Design review of the part built by this model. Coordinates are the model's own, in mm. Face numbers are marked on the shaded views. A direction names the side the tool comes from. Give positions to 0.01 mm unless a question says otherwise; leave off trailing zeros. Loops run counter-clockwise (first coordinate to the right, second up) from the corner with the lowest first, then second, coordinate; pieces in that order, holes last. Notation, with made-up numbers: (31.5, 34) -> (81.5, 34) arc R6 ccw to (81.5, 39) -> close; hole circle Ø5 at (-17, 46). An arc over 180 degrees is marked (long way). Answer in a Markdown table with one row per item. Add a question column.
(1) Consider section C-C on x = 121.5. Write out the cut boundary in (y, z).
(2) Draft analysis for pull direction Z (two halves, no side actions). For the marked faces 4, 5, 6 and 7, state which applies: +Z half, -Z half, draft (parallel to the pull), parting line (faces both ways), or undercut.
(3) Consider section B-B on z = -53. Write out the cut boundary in (x, y), then the cut area to 3 significant figures.
(4) Consider section D-D on z = -91. Write out the cut boundary in (x, y).
(5) For pin 1 (3 mm diameter, centred on x = 25, z = -34, fed in from -Y); pin 2 (4.5 mm diameter, centred on x = 77, y = -2.5, fed in from -Z); pin 3 (6.5 mm diameter, centred on x = 144, z = -50.5, fed in from +Y), all flat-tipped, find the tip position at first contact; note any pin that passes through.
(6) For the marked faces 1, 2 and 3, list the 3-axis set-ups (+Z, -Z, +X, -X, +Y, -Y) from which the entire face can be reached by the end or side of a thin tool; tool diameter is ignored.
(7) For line 1 (Y direction, x = 143.5, z = -72.5); line 2 (Z direction, x = 125.5, y = 10); line 3 (Y direction, x = 27.5, z = -44), list the stretches that pass through material, from the lowest coordinate up.
Autodesk Fusion 360 part; units mm, degrees
sketch "Sketch1" plane through (0, 0, 0) normal (0, 1, 0) x (1, 0, 0)
  line L0 (0, 0) -> (165.1, 0)
  line L1 (165.1, 0) -> (165.1, 101.6)
  line L2 (165.1, 101.6) -> (0, 101.6)
  line L3 (0, 101.6) -> (0, 0)
  dimension "d1" = 165.1
  dimension "d2" = 101.6
extrude "Extrude1" add sketch "Sketch1" along normal blind 82.55
sketch "Sketch2" plane through (165.1, 0, 0) normal (1, 0, 0) x (0, 0, -1)
  line L0 (0, 0) -> (101.6, 0)
  line L1 (101.6, 0) -> (101.6, 82.55)
  line L2 (101.6, 82.55) -> (0, 82.55)
  line L3 (0, 82.55) -> (0, 0)
  line L4 (0, 82.55) -> (0, 63.5)
  line L5 (0, 63.5) -> (19.05, 82.55)
  line L6 (0, 82.55) -> (19.05, 82.55)
  line L7 (101.6, 82.55) -> (101.6, 63.5)
  line L8 (101.6, 63.5) -> (82.55, 82.55)
  line L9 (82.55, 82.55) -> (101.6, 82.55)
  line L10 (0, 0) -> (20.6375, 0)
  line L11 (20.6375, 0) -> (80.9625, 0)
  line L12 (80.9625, 0) -> (101.6, 0)
  line L13 (20.6375, 0) -> (20.6375, 11.938)
  line L14 (20.6375, 11.938) -> (0, 11.938)
  line L15 (0, 11.938) -> (0, 0)
  line L16 (80.9625, 0) -> (80.9625, 11.938)
  line L17 (80.9625, 11.938) -> (101.6, 11.938)
  line L18 (101.6, 0) -> (101.6, 11.938)
  line L19 (80.9625, 11.938) -> (80.9625, 0)
  dimension "d5" = 45
  dimension "d6" = 45
  dimension "d7" = 20.6375
  dimension "d8" = 60.325
  dimension "d9" = 11.938
extrude "Extrude2" cut sketch "Sketch2" against normal blind 254 contours L0 L3 L10 L13 L14 L15 | L0 L1 L12 L16 L17 L18 L19 | L2 L3 L4 L5 L6 | L1 L2 L7 L8 L9
sketch "Sketch3" plane through (0, 0, 0) normal (0, -1, 0) x (1, 0, 0)
  line L0 (165.1, -20.6375) -> (0, -20.6375)
  line L1 (0, -20.6375) -> (0, -80.9625)
  line L2 (0, -80.9625) -> (165.1, -80.9625)
  line L3 (165.1, -80.9625) -> (165.1, -20.6375)
  line L4 (165.1, -20.6375) -> (165.1, -28.2575)
  line L5 (165.1, -80.9625) -> (165.1, -73.3425)
  line L6 (165.1, -28.2575) -> (152.4, -28.2575)
  line L7 (152.4, -28.2575) -> (152.4, -73.3425)
  line L8 (152.4, -73.3425) -> (165.1, -73.3425)
  line L9 (165.1, -73.3425) -> (165.1, -28.2575)
  line L10 (152.4, -50.8) -> (81.026, -50.8)
  line L11 (81.026, -50.8) -> (81.026, -35.052)
  line L12 (81.026, -50.8) -> (81.026, -66.548)
  line L13 (81.026, -35.052) -> (75.311, -35.052)
  line L14 (75.311, -35.052) -> (75.311, -66.548)
  line L15 (75.311, -66.548) -> (81.026, -66.548)
  line L16 (81.026, -66.548) -> (81.026, -35.052)
  line L17 (75.311, -50.8) -> (57.023, -50.8)
  line L18 (57.023, -50.8) -> (57.023, -31.115)
  line L19 (57.023, -50.8) -> (57.023, -70.485)
  line L20 (57.023, -70.485) -> (0, -70.485)
  line L21 (57.023, -31.115) -> (0, -31.115)
  line L22 (0, -31.115) -> (0, -70.485)
  dimension "d12" = 7.62
  dimension "d13" = 7.62
  dimension "d14" = 12.7
  dimension "d15" = 71.374
  dimension "d16" = 15.748
  dimension "d17" = 15.748
  dimension "d18" = 5.715
  dimension "d19" = 31.496
  dimension "d20" = 18.288
  dimension "d21" = 19.685
  dimension "d22" = 19.685
extrude "Extrude3" cut sketch "Sketch3" against normal up to surface (11.938 mm away) contours L3 L6 L7 L8 L9
extrude "Extrude4" add sketch "Sketch3" along normal blind 4.064 contours L11 L12 L13 L14 L15 L16
sketch "Sketch4" plane through (0, 0, -66.548) normal (0, 0, -1) x (-1, 0, 0)
  line L0 (-75.311, 0) -> (-81.026, 0)
  line L1 (-81.026, 0) -> (-81.026, -4.064)
  line L2 (-81.026, -4.064) -> (-75.311, -4.064)
  line L3 (-75.311, -4.064) -> (-75.311, 0)
  line L4 (-75.311, -4.064) -> (-81.026, 0)
  line L5 (-81.026, 0) -> (-81.026, -4.064)
  line L6 (-75.311, -4.064) -> (-81.026, -4.064)
extrude "Extrude5" cut sketch "Sketch4" against normal blind 38.1 contours L1 L2 L4 L5 L6
extrude "Extrude6" cut sketch "Sketch3" against normal blind 1.27 contours L1 L18 L19 L20 L21 L22
sketch "Sketch5" plane through (0, 0, 0) normal (-1, 0, 0) x (0, 0, 1)
  line L0 (-70.485, 0) -> (-70.485, 1.27)
  line L1 (-70.485, 1.27) -> (-31.115, 1.27)
  line L2 (-31.115, 1.27) -> (-31.115, 0)
  line L3 (-31.115, 0) -> (-20.6375, 0)
  line L4 (-20.6375, 0) -> (-20.6375, 11.938)
  line L5 (-20.6375, 11.938) -> (0, 11.938)
  line L6 (0, 11.938) -> (0, 63.5)
  line L7 (0, 63.5) -> (-19.05, 82.55)
  line L8 (-19.05, 82.55) -> (-82.55, 82.55)
  line L9 (-82.55, 82.55) -> (-101.6, 63.5)
  line L10 (-101.6, 63.5) -> (-101.6, 11.938)
  line L11 (-101.6, 11.938) -> (-80.9625, 11.938)
  line L12 (-80.9625, 11.938) -> (-80.9625, 0)
  line L13 (-80.9625, 0) -> (-70.485, 0)
  line L14 (-31.115, 1.27) -> (-70.485, 1.27)
  line L15 (-70.485, 1.27) -> (-70.485, 5.0232)
  line L16 (-70.485, 5.0232) -> (-31.115, 5.0232)
  line L17 (-31.115, 5.0232) -> (-31.115, 1.27)
extrude "Extrude7" cut sketch "Sketch5" against normal blind 1.27 contours L1 L14 L15 L16 L17
sketch "Sketch6" plane through (165.1, 0, 0) normal (1, 0, 0) x (0, 0, -1)
  line L0 (73.3425, 11.938) -> (73.3425, 0)
  line L1 (73.3425, 0) -> (80.9625, 0)
  line L2 (80.9625, 0) -> (80.9625, 11.938)
  line L3 (80.9625, 11.938) -> (101.6, 11.938)
  line L4 (101.6, 11.938) -> (101.6, 63.5)
  line L5 (101.6, 63.5) -> (82.55, 82.55)
  line L6 (82.55, 82.55) -> (19.05, 82.55)
  line L7 (19.05, 82.55) -> (0, 63.5)
  line L8 (0, 63.5) -> (0, 11.938)
  line L9 (0, 11.938) -> (20.6375, 11.938)
  line L10 (20.6375, 11.938) -> (20.6375, 0)
  line L11 (20.6375, 0) -> (28.2575, 0)
  line L12 (28.2575, 0) -> (28.2575, 11.938)
  line L13 (28.2575, 11.938) -> (73.3425, 11.938)
  line L14 (20.6375, 11.938) -> (24.7015, 11.938)
  line L15 (24.7015, 11.938) -> (24.7015, 3.048)
  line L16 (24.7015, 3.048) -> (20.6375, 3.048)
  line L17 (20.6375, 3.048) -> (20.6375, 11.938)
  line L18 (80.9625, 11.938) -> (76.8985, 11.938)
  line L19 (76.8985, 11.938) -> (76.8985, 3.048)
  line L20 (76.8985, 3.048) -> (80.9625, 3.048)
  line L21 (80.9625, 3.048) -> (80.9625, 11.938)
  dimension "d33" = 4.064
  dimension "d34" = 8.89
  dimension "d35" = 4.064
  dimension "d36" = 8.89
extrude "Extrude8" cut sketch "Sketch6" against normal blind 110.744 contours L2 L18 L19 L20 L21
extrude "Extrude9" cut sketch "Sketch6" against normal blind 110.744 contours L10 L14 L15 L16 L17
fillet "Fillet1" radius 3.81 2 edges at (165.1, 1.524, -80.9625) (165.1, 1.524, -20.6375)
sketch "Sketch7" plane through (152.4, 0, 0) normal (1, 0, 0) x (0, 0, -1)
  line L0 (73.3425, 11.938) -> (28.2575, 11.938)
  line L1 (28.2575, 11.938) -> (28.2575, 0)
  line L2 (28.2575, 0) -> (73.3425, 0)
  line L3 (73.3425, 0) -> (73.3425, 11.938)
  line L4 (73.3425, 11.938) -> (28.2575, 11.938)
  line L5 (28.2575, 11.938) -> (28.2575, 3.302)
  line L6 (28.2575, 3.302) -> (73.3425, 3.302)
  line L7 (73.3425, 3.302) -> (73.3425, 11.938)
  line L8 (73.3425, 3.302) -> (65.7225, 3.302)
  line L9 (65.7225, 3.302) -> (65.7225, 10.16)
  line L10 (65.7225, 10.16) -> (64.9605, 10.16)
  line L11 (64.9605, 10.16) -> (64.9605, 3.302)
  line L12 (64.9605, 3.302) -> (65.7225, 3.302)
  line L13 (28.2575, 3.302) -> (35.8775, 3.302)
  line L14 (35.8775, 3.302) -> (35.8775, 10.16)
  line L15 (35.8775, 10.16) -> (36.6395, 10.16)
  line L16 (36.6395, 10.16) -> (36.6395, 3.302)
  dimension "d43" = 8.636
  dimension "d44" = 7.62
  dimension "d45" = 0.762
  dimension "d46" = 7.62
  dimension "d47" = 6.858
  dimension "d48" = 0.762
extrude "Extrude10" cut sketch "Sketch7" against normal blind 12.7 contours L0 L1 L3 L4 L5 L6 L7 L8 L9 L10 L11 L13 L14 L15 L16
sketch "Sketch8" plane through (165.1, 0, 0) normal (1, 0, 0) x (0, 0, -1)
  line L0 (24.4475, 3.048) -> (24.4475, 0)
  line L1 (24.4475, 0) -> (28.2575, 0)
  line L2 (28.2575, 0) -> (28.2575, 11.938)
  line L3 (28.2575, 11.938) -> (73.3425, 11.938)
  line L4 (73.3425, 11.938) -> (73.3425, 0)
  line L5 (73.3425, 0) -> (77.1525, 0)
  line L6 (77.1525, 0) -> (77.1525, 3.048)
  line L7 (77.1525, 3.048) -> (76.8985, 3.048)
  line L8 (76.8985, 3.048) -> (76.8985, 11.938)
  line L9 (76.8985, 11.938) -> (101.6, 11.938)
  line L10 (101.6, 11.938) -> (101.6, 63.5)
  line L11 (101.6, 63.5) -> (82.55, 82.55)
  line L12 (82.55, 82.55) -> (19.05, 82.55)
  line L13 (19.05, 82.55) -> (0, 63.5)
  line L14 (0, 63.5) -> (0, 11.938)
  line L15 (0, 11.938) -> (24.7015, 11.938)
  line L16 (24.7015, 11.938) -> (24.7015, 3.048)
  line L17 (24.7015, 3.048) -> (24.4475, 3.048)
  line L18 (50.8, 82.55) -> (63.5, 82.55)
  line L19 (50.8, 82.55) -> (38.1, 82.55)
  line L20 (38.1, 82.55) -> (38.1, 81.28)
  line L21 (38.1, 81.28) -> (63.5, 81.28)
  line L22 (63.5, 81.28) -> (63.5, 82.55)
  dimension "d51" = 1.27
extrude "Extrude11" cut sketch "Sketch8" against normal blind 144.78 contours L12 L18 L19 L20 L21 L22
sketch "Sketch9" plane through (0, 81.28, 0) normal (0, 1, 0) x (-1, 0, 0)
  line L0 (-165.1, -38.1) -> (-165.1, -63.5)
  line L1 (-165.1, -63.5) -> (-20.32, -63.5)
  line L2 (-20.32, -63.5) -> (-20.32, -38.1)
  line L3 (-20.32, -38.1) -> (-165.1, -38.1)
chamfer "Chamfer2" distance 7.62 angle 45 6 edges at (165.1, 82.55, -73.025) (165.1, 73.025, -92.075) (165.1, 37.719, -101.6) (165.1, 82.55, -28.575) (165.1, 73.025, -9.525) (165.1, 37.719, 0)
chamfer "Chamfer3" distance 7.62 angle 45 5 edges at (0, 37.719, -101.6) (0, 73.025, -92.075) (0, 82.55, -50.8) (0, 73.025, -9.525) (0, 37.719, 0)
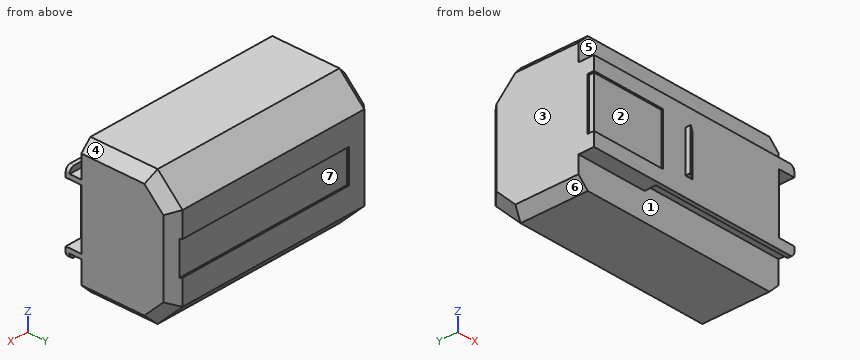
Values follow:
| question | item | result |
|---|---|---|
| 1 | outline | (0, -80.96) -> (3.05, -80.96) -> (3.05, -76.9) -> (11.94, -76.9) -> (11.94, -101.6) -> (63.5, -101.6) -> (82.55, -82.55) -> (82.55, -63.5) -> (81.28, -63.5) -> (81.28, -38.1) -> (82.55, -38.1) -> (82.55, -19.05) -> (63.5, 0) -> (11.94, 0) -> (11.94, -24.7) -> (3.05, -24.7) -> (3.05, -20.64) -> (0, -20.64) -> close |
| 2 | face 4 | +Z half |
| 2 | face 5 | draft |
| 2 | face 6 | -Z half |
| 2 | face 7 | undercut |
| 3 | outline | (0, 5.02) -> (1.27, 5.02) -> (1.27, 1.27) -> (57.02, 1.27) -> (57.02, 0) -> (75.31, 0) -> (75.31, -4.06) -> (81.03, 0) -> (152.4, 0) -> (152.4, 3.3) -> (139.7, 3.3) -> (139.7, 11.94) -> (165.1, 11.94) -> (165.1, 74.93) -> (158.75, 81.28) -> (20.32, 81.28) -> (20.32, 82.55) -> (7.62, 82.55) -> (0, 74.93) -> close |
| 3 | area | 13,100 mm2 |
| 4 | outline | (0, 11.94) -> (165.1, 11.94) -> (165.1, 63.32) -> (157.48, 74.1) -> (7.62, 74.1) -> (0, 63.32) -> close |
| 5 | pin 1 | y = 1.27 |
| 5 | pin 2 | z = -66.55 |
| 5 | pin 3 | y = 81.28 |
| 6 | face 1 | -Z, +X |
| 6 | face 2 | -X, -Y |
| 6 | face 3 | +Z, -Z, -X, +Y, -Y |
| 7 | line 1 | 0 to 3.3, 11.94 to 82.55 |
| 7 | line 2 | -76.9 to -24.7 |
| 7 | line 3 | 1.27 to 81.28 |
